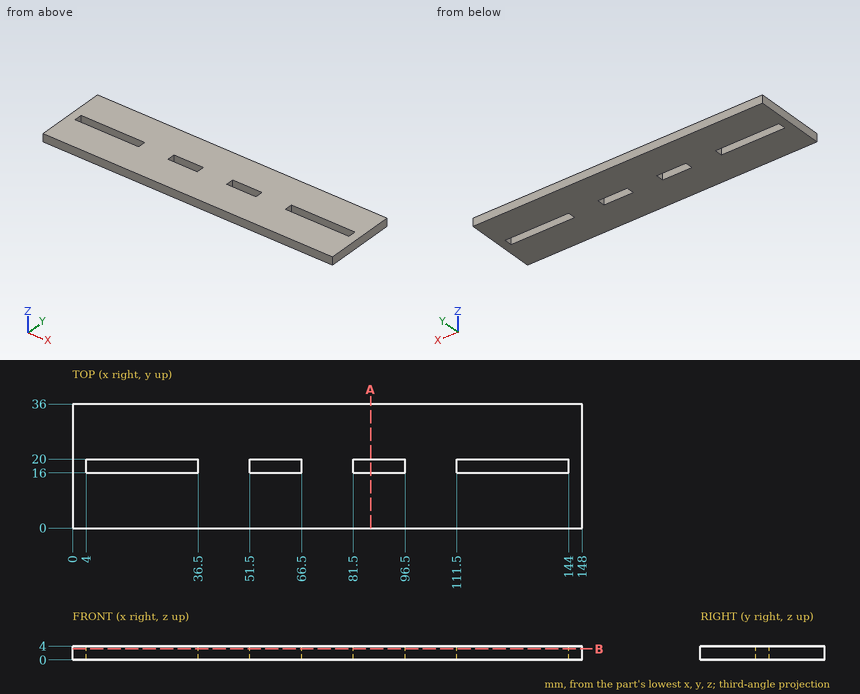
The figure shows three views and two pictorial views of one solid part (mm, origin at its lowest corner). Answer the questions. Round coordinates to 2 decimals unless told otherwise and drop trailing zeros. Order: outer loops, then holes, each group sorted by start corner. A loop starts at its lowest first (then second) coordinate and runs counter-clockwise, first axis right, second up. Notation, with made-up numbers: (70, 27.25) -> (74, 27.25) arc R20 cw to (74, 40.25) -> close; hole circle Ø10 at (39, 44). An arc over 180 degrees is marked (long way). Put each result on its own line as item: value.
Q1. Section A-A, the plane x = 86.5 is taken. Write down the section's boundary in (y, z).
Results list:
outline: (0, 0) -> (16, 0) -> (16, 4) -> (0, 4) -> close; (20, 0) -> (36, 0) -> (36, 4) -> (20, 4) -> close
Q2. Section B-B, the plane z = 3.2 is taken. Write down the section's boundary in (x, y), and give its area (3 significant figures).
Results list:
outline: (0, 0) -> (148, 0) -> (148, 36) -> (0, 36) -> close; hole (4, 16) -> (36.5, 16) -> (36.5, 20) -> (4, 20) -> close; hole (51.5, 16) -> (66.5, 16) -> (66.5, 20) -> (51.5, 20) -> close; hole (81.5, 16) -> (96.5, 16) -> (96.5, 20) -> (81.5, 20) -> close; hole (111.5, 16) -> (144, 16) -> (144, 20) -> (111.5, 20) -> close
area: 4,950 mm^2
Q3. Consider line 1 along X through (y, z) = (19, 1.5); line 2 along Y through (x, z) = (9, 2.95). Determine where each line is inside the solid, lowest interval first.
Results list:
line 1: 0 to 4, 36.5 to 51.5, 66.5 to 81.5, 96.5 to 111.5, 144 to 148
line 2: 0 to 16, 20 to 36
